Input: part model. Units: mm. Frame: model coordinates. Round coordinates to 2 decimals unless told otherwise and drop trailing zeros. Order: outer loops, then holes, each group sorted by start corner. A loop starts at its lowest first (then second) coordinate and runs counter-clockwise, first axis right, second up.
Item 1: Cut plane B-B on y = -25.5. Output: boundary loops of the cut face in (x, z).
Item 2: Cut plane A-A on x = 5. Give the number of separate pieces and of enclosed holes in the cut face, then the cut area to 3 significant figures.
Item 3: Line query: L1, parallel to Z at x = 5, y = -50.8 (3 decimals); L2, parallel to Y at x = 5, z = 0 (3 decimals); L3, parallel to Z at x = 3, y = 74. Output: solid intervals per line, ascending.
Item 4: First-contact query: pin 1 (1.9 mm diameter, centred on x = 2, y = -177, fed in from +Z); pin 2 (3 mm diameter, centred on x = 2.5, y = -432.5, fed in from -Z); pin 3 (2 mm diameter, centred on x = 3, z = 9, fed in from -Y). Flat tips, straight axial feed; report the tip coordinate or a pass-through.
Item 5: Cut plane C-C on z = 66.5. Output: boundary loops of the cut face in (x, y).
Autodesk Inventor part; units mm, degrees
ref_plane "YZ Plane" through (0, 0, 0) normal (1, 0, 0) x (0, 1, 0)
ref_plane "XZ Plane" through (0, 0, 0) normal (0, 1, 0) x (-1, 0, 0)
ref_plane "XY Plane" through (0, 0, 0) normal (0, 0, 1) x (1, 0, 0)
sketch "Sketch1" plane through (0, 0, 0) normal (1, 0, 0) x (0, 1, 0)
  circle A0 centre (0, 0) radius 3.175
  line L0 (0, 0) -> (12.7, 0)
  line L1 (0, 0) -> (12.7, 0) construction
  line L2 (12.7, 0) -> (12.7, -12.7)
  line L3 (12.7, -12.7) -> (-405.9936, -12.7)
  line L4 (-405.9936, -12.7) -> (-405.9936, 12.7)
  line L5 (-405.9936, 12.7) -> (12.7, 12.7)
  line L6 (12.7, 12.7) -> (12.7, -12.7)
  line L7 (-405.9936, 12.7) -> (-498.3106, 105.017)
  line L8 (-405.9936, 12.7) -> (-275.4376, 12.7) construction
  line L9 (-498.3106, 105.017) -> (-516.2711, 87.0565)
  line L10 (-516.2711, 87.0565) -> (-408.5081, -20.7066)
  line L11 (-405.9936, -12.7) -> (-431.3936, -12.7)
  line L12 (-405.9936, -12.7) -> (-380.5936, -12.7) construction
  line L13 (-516.2711, 87.0565) -> (-416.5146, -12.7)
  line L14 (-416.5146, -12.7) -> (12.7, -12.7)
  dimension "d0" = 6.35
  dimension "d1" = 12.7
  dimension "d2" = 0
  dimension "d3" = 12.7
  dimension "d4" = 90
  dimension "d5" = 418.6936
  dimension "d6" = 25.4
  dimension "d7" = 130.556
  dimension "d8" = 135
  dimension "d9" = 25.4
  dimension "d10" = 90
  dimension "d11" = 152.4
  dimension "d12" = 90
  dimension "d13" = 25.4
  dimension "d14" = 180
extrude "Extrusion1" add sketch "Sketch1" along normal blind 25.4
sketch "Sketch2" plane through (25.4, 0, 0) normal (1, 0, 0) x (0, 0, -1)
  line L0 (-105.017, -498.3106) -> (-87.0565, -516.2711)
  line L1 (-87.0565, -516.2711) -> (12.7, -416.5146)
  line L2 (-12.7, 12.7) -> (-12.7, -405.9936)
  line L3 (-96.0368, -507.2909) -> (-78.0763, -507.2909)
  line L4 (-105.017, -498.3106) -> (-100.5269, -502.8008)
  line L5 (-100.5269, -502.8008) -> (-73.5861, -502.8008)
  arc A0 (-100.5269, -502.8008) -> (-73.5861, -502.8008) centre (-87.0565, -489.3304) ccw
  dimension "d17" = 6.35
  dimension "d18" = 19.05
extrude "Extrusion2" cut sketch "Sketch2" against normal blind 25.4 contours A0 L3 L0 | L3 A0 L1 L0 | L1 L3 A0
sketch "Sketch3" plane through (0, 12.7, 12.7) normal (0, 1, 0) x (1, 0, 0)
  line L0 (0, 25.4) -> (0, 0)
  line L1 (0, 0) -> (25.4, 0)
  line L2 (25.4, 25.4) -> (25.4, 0)
  line L3 (0, 25.4) -> (25.4, 25.4)
  point P0 (0, 12.7)
extrude "Extrusion3" add sketch "Sketch3" along normal blind 127
sketch "Sketch4" plane through (25.4, 0, 0) normal (1, 0, 0) x (0, 0, -1)
  arc A0 (-100.5269, -502.8008) -> (-73.5861, -502.8008) centre (-87.0565, -489.3304) ccw
  line L0 (-73.5861, -502.8008) -> (12.7, -416.5146)
  line L1 (12.7, -416.5146) -> (12.7, 139.7)
  line L2 (-12.7, 139.7) -> (12.7, 139.7)
  line L3 (-12.7, -405.9936) -> (-12.7, 139.7)
  line L4 (-12.7, -405.9936) -> (-105.017, -498.3106)
  line L5 (-105.017, -498.3106) -> (-100.5269, -502.8008)
  circle A1 centre (0, 0) radius 3.175
extrude "Extrusion4" cut sketch "Sketch4" against normal blind 19.05
sketch "Sketch5" plane through (6.35, 0, 0) normal (1, 0, 0) x (0, 0, -1)
  line L0 (-12.7, 139.7) -> (12.7, 139.7)
  line L1 (12.7, 139.7) -> (12.7, 12.7)
  line L2 (12.7, 12.7) -> (-12.7, 12.7)
  line L3 (-12.7, 12.7) -> (-12.7, 139.7)
  dimension "d25" = 25.4
  dimension "d26" = 127
extrude "Extrusion5" cut sketch "Sketch5" against normal blind 127
sketch "Sketch8" plane through (6.35, 12.7, 12.7) normal (0, 1, 0) x (1, 0, 0)
  line L0 (-6.35, 0) -> (-6.35, 25.4)
  line L1 (0, 0) -> (-6.35, 0)
  line L2 (0, 25.4) -> (0, 0)
  line L3 (-6.35, 25.4) -> (0, 25.4)
  point P0 (-6.35, 12.7)
extrude "Extrusion8" add sketch "Sketch8" along normal blind 101.6
sketch "Sketch9" plane through (6.35, 0, 0) normal (1, 0, 0) x (0, 0, -1)
  circle A0 centre (0, 0) radius 3.175
  circle A1 centre (0, 0) radius 6.35
  dimension "d45" = 12.7
extrude "Extrusion9" cut sketch "Sketch9" against normal blind 25.4
sketch "Sketch10" plane through (6.35, 0, 0) normal (1, 0, 0) x (0, 0, -1)
  circle A0 centre (0, 0) radius 6.35
  line L0 (0, 6.35) -> (5.4993, 3.175)
  line L1 (5.4993, 3.175) -> (5.4993, -3.175)
  line L2 (5.4993, -3.175) -> (0, -6.35)
  line L3 (0, -6.35) -> (-5.4993, -3.175)
  line L4 (-5.4993, -3.175) -> (-5.4993, 3.175)
  line L5 (-5.4993, 3.175) -> (0, 6.35)
extrude "Extrusion11" add sketch "Sketch10" against normal blind 6.35 contours A0 L1 | L0 A0 | A0 L2 | L5 A0 | A0 L3 | L4 A0
sketch "Sketch11" plane through (6.35, 0, 0) normal (1, 0, 0) x (0, 0, -1)
  line L0 (12.7, 114.3) -> (12.7, -416.5146)
  line L1 (-12.7, 114.3) -> (12.7, 114.3)
  line L2 (0, 114.3) -> (0, 50.8)
  line L3 (0, 114.3) -> (63.5, 114.3) construction
  line L4 (0, 50.8) -> (0, -50.8)
  line L5 (0, 50.8) -> (101.6, 50.8) construction
  circle A0 centre (0, 50.8) radius 3.175
  circle A1 centre (0, -50.8) radius 3.175
  point P0 (0, 0)
  dimension "d54" = 63.5
  dimension "d55" = 90
  dimension "d56" = 101.6
  dimension "d57" = 90
  dimension "d58" = 6.35
  dimension "d59" = 6.35
extrude "Extrusion12" cut sketch "Sketch11" against normal blind 6.35
properties part number "FlatArm"
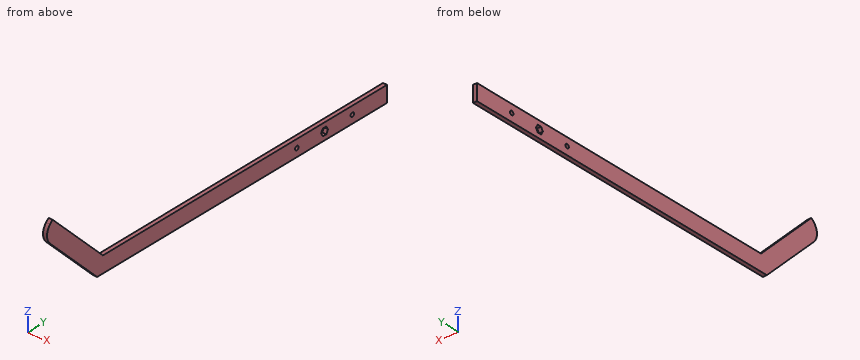
From the geometry:
1. outline: (0, -12.7) - (6.35, -12.7) - (6.35, 12.7) - (0, 12.7) - close
2. separate pieces: 1
2. enclosed holes: 3
2. area: 16,600 mm2
3. L1: z = -12.7 to -3.175, 3.175 to 12.7
3. L2: y = -429.215 to -53.975, -47.625 to -6.35, 6.35 to 47.625, 53.975 to 114.3
3. L3: z = -12.7 to 12.7
4. pin 1: stops at z = 12.7
4. pin 2: stops at z = 1.79
4. pin 3: stops at y = -439.21
5. outline: (0, -495.71) - (6.35, -495.71) - (6.35, -459.79) - (0, -459.79) - close
